Source: CAD feature listing. Evaluate the final solid. Frame: model axes, mm. Face numbers are marked on the shaded views. A direction names the side the tool comes from. Give positions to 0.01 mm unless a question says otherwise; leave off trailing zeros. Write each loop counter-clockwise with the first axis right and the second up, starting at its lowest first coordinate (ties: lowest second). Pieces come first, ordered by that corner, then holes. Notation, with made-up numbers: (87, -40) -> (121, -40) arc R15 ccw to (121, -17) -> close; hole circle Ø2 at (-12, -4.75). An arc over 180 degrees is marked (long way). Use a Markdown table: item, result. Add a question column.
```python
from build123d import *

# Parameters (mm, degrees)
EXTRUDE_1_DEPTH      = 7.5
EXTRUDE_1_DEPTH_BACK = 7.5
SKETCH_1_W           = 60
SKETCH_1_H           = 15
SKETCH_2_W           = 3
SKETCH_2_H           = 3
EXTRUDE_2_DEPTH      = 1
EXTRUDE_3_DEPTH      = 1
EXTRUDE_3_DEPTH_BACK = 4
CUT_EXTRUDE_1_REACH  = 36.667
SKETCH_5_W           = 54.5
SKETCH_5_H           = 13
CUT_EXTRUDE_2_DEPTH  = 13
CUT_EXTRUDE_3_DEPTH  = 9.45
EXTRUDE_4_REACH      = 40.81
SKETCH_7_W           = 0.3
SKETCH_7_H           = 6.5
CUT_EXTRUDE_4_REACH  = 40.082
CUT_EXTRUDE_5_REACH  = 37.798
FILLET_1_R           = 0.1
FILLET_2_R           = 0.2


with BuildPart() as part:
    # Sketch 1 → Extrude 1 (new, two sides: drawn at the far end of the back side and taken through both)
    with BuildSketch(Plane.XY.offset(-EXTRUDE_1_DEPTH_BACK)):
        with Locations((0, 7.5)):
            Rectangle(SKETCH_1_W, SKETCH_1_H)
    extrude(amount=EXTRUDE_1_DEPTH + EXTRUDE_1_DEPTH_BACK)

    # Sketch 2 → Extrude 2 (add)
    with BuildSketch(Plane(origin=(30, 0, 0), x_dir=(0, 0, -1), z_dir=(1, 0, 0))):
        with Locations((0, 7.5)):
            Rectangle(SKETCH_2_W, SKETCH_2_H)
    extrude(amount=EXTRUDE_2_DEPTH)

    # Sketch 3 → Extrude 3 (add, two sides: drawn at the far end of the back side and taken through both)
    with BuildSketch(Plane.XY.offset(1.5).offset(-EXTRUDE_3_DEPTH_BACK)):
        with BuildLine():
            Line((32.5, 9.45), (32.5, 5.55))
            Line((32.5, 5.55), (31.555590279, 5.55))
            ThreePointArc((31.555590279, 5.55), (31.088161527, 5.719957697), (30.677124344, 6))
            Line((30.677124344, 6), (30.677124344, 9))
            ThreePointArc((30.677124344, 9), (31.088161527, 9.280042303), (31.555590279, 9.45))
            Line((31.555590279, 9.45), (32.5, 9.45))
        make_face()
    extrude(amount=EXTRUDE_3_DEPTH + EXTRUDE_3_DEPTH_BACK)

    # Sketch 4 → Cut-Extrude 1 (cut, up to next)
    with BuildSketch(Plane(origin=(0, 9.45, 0), x_dir=(-1, 0, 0), z_dir=(0, 1, 0)), mode=Mode.PRIVATE) as cut_extrude_1_sk1:
        with BuildLine():
            Line((-32.5, -1.95), (-31.555590279, -1.95))
            ThreePointArc((-31.555590279, -1.95), (-31.088161527, -1.780042303), (-30.677124344, -1.5))
            Line((-30.677124344, -1.5), (-30.677124344, -2.5))
            Line((-30.677124344, -2.5), (-32.5, -2.5))
            Line((-32.5, -2.5), (-32.5, -1.95))
        make_face()
    cut_extrude_1_tool1 = extrude(cut_extrude_1_sk1.sketch, amount=-CUT_EXTRUDE_1_REACH, mode=Mode.PRIVATE) & part.part
    # Sketch 4 → Cut-Extrude 1 (cut, up to next)
    with BuildSketch(Plane(origin=(0, 9.45, 0), x_dir=(-1, 0, 0), z_dir=(0, 1, 0)), mode=Mode.PRIVATE) as cut_extrude_1_sk2:
        with BuildLine():
            Line((-30.677124344, 2.5), (-32.5, 2.5))
            Line((-32.5, 2.5), (-32.5, 1.95))
            Line((-32.5, 1.95), (-31.555590279, 1.95))
            ThreePointArc((-31.555590279, 1.95), (-31.088161527, 1.780042303), (-30.677124344, 1.5))
            Line((-30.677124344, 1.5), (-30.677124344, 2.5))
        make_face()
    cut_extrude_1_tool2 = extrude(cut_extrude_1_sk2.sketch, amount=-CUT_EXTRUDE_1_REACH, mode=Mode.PRIVATE) & part.part
    add(cut_extrude_1_tool1.solids().sort_by_distance((31.500125, 9.45, -2.169375))[0], mode=Mode.SUBTRACT)
    add(cut_extrude_1_tool2.solids().sort_by_distance((31.500125, 9.45, 2.169375))[0], mode=Mode.SUBTRACT)

    # Sketch 5 → Cut-Extrude 2 (cut)
    with BuildSketch(Plane.XY.offset(7.5)):
        with Locations((0.75, 8.5)):
            Rectangle(SKETCH_5_W, SKETCH_5_H)
    extrude(amount=-CUT_EXTRUDE_2_DEPTH, mode=Mode.SUBTRACT)

    # Sketch 6 → Cut-Extrude 3 (cut)
    with BuildSketch(Plane.XY.offset(7.5)):
        with BuildLine():
            Line((-27.2, 9.45), (-27.2, 5.55))
            Line((-27.2, 5.55), (-28.444409721, 5.55))
            ThreePointArc((-28.444409721, 5.55), (-28.911838473, 5.719957697), (-29.322875656, 6))
            Line((-29.322875656, 6), (-30, 6))
            Line((-30, 6), (-30, 9))
            Line((-30, 9), (-29.322875656, 9))
            ThreePointArc((-29.322875656, 9), (-28.911838473, 9.280042303), (-28.444409721, 9.45))
            Line((-28.444409721, 9.45), (-27.2, 9.45))
        make_face()
    extrude(amount=-CUT_EXTRUDE_3_DEPTH, mode=Mode.SUBTRACT)

    # Sketch 7 → Extrude 4 (add, up to next)
    with BuildSketch(Plane.XY.offset(7.5), mode=Mode.PRIVATE) as extrude_4_sk1:
        with Locations((-26.35, 7.5)):
            Rectangle(SKETCH_7_W, SKETCH_7_H)
    extrude_4_tool1 = extrude(extrude_4_sk1.sketch, amount=-EXTRUDE_4_REACH, mode=Mode.PRIVATE) - part.part
    add(extrude_4_tool1.solids().sort_by_distance((-26.35, 7.5, 7.5))[0])

    # Sketch 8 → Cut-Extrude 4 (cut, up to next)
    with BuildSketch(Plane.XY.offset(-5.5), mode=Mode.PRIVATE) as cut_extrude_4_sk1:
        with BuildLine():
            Line((-21.177124344, 9), (-19.25, 9))
            Line((-19.25, 9), (-19.25, 6))
            Line((-19.25, 6), (-21.177124344, 6))
            ThreePointArc((-21.177124344, 6), (-22.5, 5.5), (-23.822875656, 6))
            Line((-23.822875656, 6), (-25.75, 6))
            Line((-25.75, 6), (-25.75, 9))
            Line((-25.75, 9), (-23.822875656, 9))
            ThreePointArc((-23.822875656, 9), (-22.5, 9.5), (-21.177124344, 9))
        make_face()
    cut_extrude_4_tool1 = extrude(cut_extrude_4_sk1.sketch, amount=-CUT_EXTRUDE_4_REACH, mode=Mode.PRIVATE) & part.part
    # Sketch 8 → Cut-Extrude 4 (cut, up to next)
    with BuildSketch(Plane.XY.offset(-5.5), mode=Mode.PRIVATE) as cut_extrude_4_sk2:
        with BuildLine():
            Line((-10.75, 9), (-8.822875656, 9))
            ThreePointArc((-8.822875656, 9), (-7.5, 9.5), (-6.177124344, 9))
            Line((-6.177124344, 9), (-4.25, 9))
            Line((-4.25, 9), (-4.25, 6))
            Line((-4.25, 6), (-6.177124344, 6))
            ThreePointArc((-6.177124344, 6), (-7.5, 5.5), (-8.822875656, 6))
            Line((-8.822875656, 6), (-10.75, 6))
            Line((-10.75, 6), (-10.75, 9))
        make_face()
    cut_extrude_4_tool2 = extrude(cut_extrude_4_sk2.sketch, amount=-CUT_EXTRUDE_4_REACH, mode=Mode.PRIVATE) & part.part
    # Sketch 8 → Cut-Extrude 4 (cut, up to next)
    with BuildSketch(Plane.XY.offset(-5.5), mode=Mode.PRIVATE) as cut_extrude_4_sk3:
        with BuildLine():
            Line((6.177124344, 6), (4.25, 6))
            Line((4.25, 6), (4.25, 9))
            Line((4.25, 9), (6.177124344, 9))
            ThreePointArc((6.177124344, 9), (7.5, 9.5), (8.822875656, 9))
            Line((8.822875656, 9), (10.75, 9))
            Line((10.75, 9), (10.75, 6))
            Line((10.75, 6), (8.822875656, 6))
            ThreePointArc((8.822875656, 6), (7.5, 5.5), (6.177124344, 6))
        make_face()
    cut_extrude_4_tool3 = extrude(cut_extrude_4_sk3.sketch, amount=-CUT_EXTRUDE_4_REACH, mode=Mode.PRIVATE) & part.part
    # Sketch 8 → Cut-Extrude 4 (cut, up to next)
    with BuildSketch(Plane.XY.offset(-5.5), mode=Mode.PRIVATE) as cut_extrude_4_sk4:
        with BuildLine():
            Line((21.177124344, 6), (19.25, 6))
            Line((19.25, 6), (19.25, 9))
            Line((19.25, 9), (21.177124344, 9))
            ThreePointArc((21.177124344, 9), (22.5, 9.5), (23.822875656, 9))
            Line((23.822875656, 9), (25.75, 9))
            Line((25.75, 9), (25.75, 6))
            Line((25.75, 6), (23.822875656, 6))
            ThreePointArc((23.822875656, 6), (22.5, 5.5), (21.177124344, 6))
        make_face()
    cut_extrude_4_tool4 = extrude(cut_extrude_4_sk4.sketch, amount=-CUT_EXTRUDE_4_REACH, mode=Mode.PRIVATE) & part.part
    add(cut_extrude_4_tool1.solids().sort_by_distance((-22.5, 7.5, -5.5))[0], mode=Mode.SUBTRACT)
    add(cut_extrude_4_tool2.solids().sort_by_distance((-7.5, 7.5, -5.5))[0], mode=Mode.SUBTRACT)
    add(cut_extrude_4_tool3.solids().sort_by_distance((7.5, 7.5, -5.5))[0], mode=Mode.SUBTRACT)
    add(cut_extrude_4_tool4.solids().sort_by_distance((22.5, 7.5, -5.5))[0], mode=Mode.SUBTRACT)

    # Sketch 9 → Cut-Extrude 5 (cut, up to next)
    with BuildSketch(Plane(origin=(0, 2, 0), x_dir=(-1, 0, 0), z_dir=(0, 1, 0)), mode=Mode.PRIVATE) as cut_extrude_5_sk1:
        with BuildLine():
            Line((21.177124344, -1.5), (19.25, -1.5))
            Line((19.25, -1.5), (19.25, 1.5))
            Line((19.25, 1.5), (21.177124344, 1.5))
            ThreePointArc((21.177124344, 1.5), (22.5, 2), (23.822875656, 1.5))
            Line((23.822875656, 1.5), (25.75, 1.5))
            Line((25.75, 1.5), (25.75, -1.5))
            Line((25.75, -1.5), (23.822875656, -1.5))
            ThreePointArc((23.822875656, -1.5), (22.5, -2), (21.177124344, -1.5))
        make_face()
    cut_extrude_5_tool1 = extrude(cut_extrude_5_sk1.sketch, amount=-CUT_EXTRUDE_5_REACH, mode=Mode.PRIVATE) & part.part
    # Sketch 9 → Cut-Extrude 5 (cut, up to next)
    with BuildSketch(Plane(origin=(0, 2, 0), x_dir=(-1, 0, 0), z_dir=(0, 1, 0)), mode=Mode.PRIVATE) as cut_extrude_5_sk2:
        with BuildLine():
            Line((10.75, -1.5), (8.822875656, -1.5))
            ThreePointArc((8.822875656, -1.5), (7.5, -2), (6.177124344, -1.5))
            Line((6.177124344, -1.5), (4.25, -1.5))
            Line((4.25, -1.5), (4.25, 1.5))
            Line((4.25, 1.5), (6.177124344, 1.5))
            ThreePointArc((6.177124344, 1.5), (7.5, 2), (8.822875656, 1.5))
            Line((8.822875656, 1.5), (10.75, 1.5))
            Line((10.75, 1.5), (10.75, -1.5))
        make_face()
    cut_extrude_5_tool2 = extrude(cut_extrude_5_sk2.sketch, amount=-CUT_EXTRUDE_5_REACH, mode=Mode.PRIVATE) & part.part
    # Sketch 9 → Cut-Extrude 5 (cut, up to next)
    with BuildSketch(Plane(origin=(0, 2, 0), x_dir=(-1, 0, 0), z_dir=(0, 1, 0)), mode=Mode.PRIVATE) as cut_extrude_5_sk3:
        with BuildLine():
            Line((-6.177124344, 1.5), (-4.25, 1.5))
            Line((-4.25, 1.5), (-4.25, -1.5))
            Line((-4.25, -1.5), (-6.177124344, -1.5))
            ThreePointArc((-6.177124344, -1.5), (-7.5, -2), (-8.822875656, -1.5))
            Line((-8.822875656, -1.5), (-10.75, -1.5))
            Line((-10.75, -1.5), (-10.75, 1.5))
            Line((-10.75, 1.5), (-8.822875656, 1.5))
            ThreePointArc((-8.822875656, 1.5), (-7.5, 2), (-6.177124344, 1.5))
        make_face()
    cut_extrude_5_tool3 = extrude(cut_extrude_5_sk3.sketch, amount=-CUT_EXTRUDE_5_REACH, mode=Mode.PRIVATE) & part.part
    # Sketch 9 → Cut-Extrude 5 (cut, up to next)
    with BuildSketch(Plane(origin=(0, 2, 0), x_dir=(-1, 0, 0), z_dir=(0, 1, 0)), mode=Mode.PRIVATE) as cut_extrude_5_sk4:
        with BuildLine():
            Line((-21.177124344, 1.5), (-19.25, 1.5))
            Line((-19.25, 1.5), (-19.25, -1.5))
            Line((-19.25, -1.5), (-21.177124344, -1.5))
            ThreePointArc((-21.177124344, -1.5), (-22.5, -2), (-23.822875656, -1.5))
            Line((-23.822875656, -1.5), (-25.75, -1.5))
            Line((-25.75, -1.5), (-25.75, 1.5))
            Line((-25.75, 1.5), (-23.822875656, 1.5))
            ThreePointArc((-23.822875656, 1.5), (-22.5, 2), (-21.177124344, 1.5))
        make_face()
    cut_extrude_5_tool4 = extrude(cut_extrude_5_sk4.sketch, amount=-CUT_EXTRUDE_5_REACH, mode=Mode.PRIVATE) & part.part
    add(cut_extrude_5_tool1.solids().sort_by_distance((-22.5, 2, 0))[0], mode=Mode.SUBTRACT)
    add(cut_extrude_5_tool2.solids().sort_by_distance((-7.5, 2, 0))[0], mode=Mode.SUBTRACT)
    add(cut_extrude_5_tool3.solids().sort_by_distance((7.5, 2, 0))[0], mode=Mode.SUBTRACT)
    add(cut_extrude_5_tool4.solids().sort_by_distance((22.5, 2, 0))[0], mode=Mode.SUBTRACT)

    # Fillet 1
    fillet_1_edges = [part.edges().sort_by_distance(p)[0] for p in [
        (32.5, 5.55, 0),
        (32.5, 9.45, 0),
        (32.5, 7.5, -1.95),
        (32.5, 7.5, 1.95),
    ]]
    fillet(fillet_1_edges, radius=FILLET_1_R)

    # Fillet 2
    fillet_2_edges = [part.edges().sort_by_distance(p)[0] for p in [
        (-30, 3, 7.5),
        (-30, 0, 0),
        (-30, 7.5, -7.5),
        (-30, 15, 0),
        (-30, 12, 7.5),
        (-30, 9, 2.775),
        (-30, 7.5, -1.95),
        (-30, 6, 2.775),
        (0, 0, -7.5),
        (0, 0, 7.5),
        (0, 15, -7.5),
        (30, 0, 0),
        (30, 7.5, -7.5),
        (30, 15, 0),
        (29, 15, 7.5),
        (30, 7.5, 7.5),
    ]]
    fillet(fillet_2_edges, radius=FILLET_2_R)


solid = part.part
```
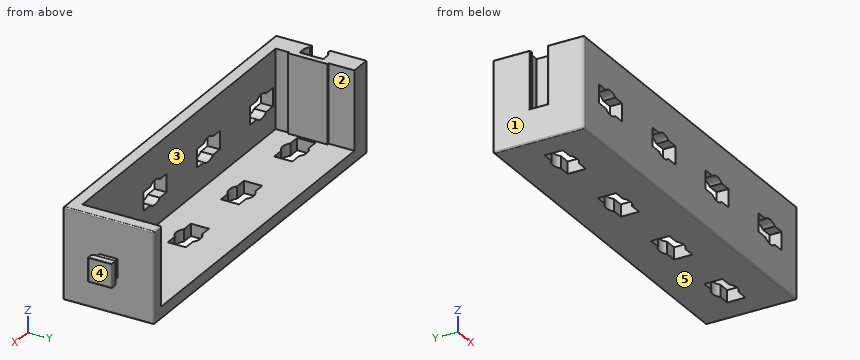
(1) Material intervals for L1, parallel to X at y = 8.25, z = -5.75; L2, parallel to X at y = 5.5, z = 4.25; L3, parallel to X at y = 11, z = 1.75, sorted ascending.
(2) Cut plane C-C on y = 12.5. Return the cut outline in (x, z), then the cut area to 3 significant figures.
(3) First-contact query: pin 1 Ø6 at (y, z) = (7, 2) entering from +X; pin 2 Ø4 at (y, z) = (12.5, -0.5) entering from +X; pin 3 Ø1 at (x, y) = (1, 4.5) entering from +Z. Flat tips, straight axial feed; report the tip coordinate or a pass-through.
(4) Cut plane B-B on z = 3.25. Return the cut outline in (x, y).
(5) Access query for the marked faces 1 and 2. Directions: +Z, -Z, +X, -X, +Y, -Y. A direction counts if a zero-diameter tool reaches every point of the face in a straight line with its end or side. Return the directions, or none.
(6) Mould query, pull axis X, two halves, no side actions, for the marked faces 3, 4 and 5. Classes: +X half, -X half, draft (parallel to the pull), parting line (faces both ways), or undercut.
(7) Cut plane A-A on x = -20. Return the cut outline in (y, z), then the cut area to 3 significant figures.
(8) Cut plane D-D on y = 6.75. Count the separate pieces of the cut face and the enclosed holes in it, then the cut area to 3 significant figures.
Output:
| question | item | result |
|---|---|---|
| 1 | L1 | -30 to -25.75, -19.25 to -10.75, -4.25 to 4.25, 10.75 to 19.25, 25.75 to 30 |
| 1 | L2 | -30 to -26.2, 28 to 30 |
| 1 | L3 | -30 to -26.5, 28 to 30 |
| 2 | outline | (-30, -7.3) arc R0.2 ccw to (-29.8, -7.5) -> (29.8, -7.5) arc R0.2 ccw to (30, -7.3) -> (30, 7.3) arc R0.2 ccw to (29.8, 7.5) -> (28, 7.5) -> (28, -5.5) -> (-26.5, -5.5) -> (-26.5, 7.5) -> (-29.8, 7.5) arc R0.2 ccw to (-30, 7.3) -> close |
| 2 | area | 191 mm^2 |
| 3 | pin 1 | x = 32.5 |
| 3 | pin 2 | x = 30 |
| 3 | pin 3 | z = -5.5 |
| 4 | outline | (-30, 0.2) arc R0.2 ccw to (-29.8, 0) -> (29.8, 0) arc R0.2 ccw to (30, 0.2) -> (30, 14.8) arc R0.2 ccw to (29.8, 15) -> (28, 15) -> (28, 2) -> (-26.5, 2) -> (-26.5, 4.25) -> (-26.2, 4.25) -> (-26.2, 10.75) -> (-26.5, 10.75) -> (-26.5, 15) -> (-29.8, 15) arc R0.2 ccw to (-30, 14.8) -> (-30, 9.2) arc R0.2 ccw to (-29.8, 9) -> (-29.32, 9) arc R2 cw to (-28.44, 9.45) -> (-27.2, 9.45) -> (-27.2, 5.55) -> (-28.44, 5.55) arc R2 cw to (-29.32, 6) -> (-29.8, 6) arc R0.2 ccw to (-30, 5.8) -> close |
| 5 | face 1 | +Z, -Z, -X, +Y, -Y |
| 5 | face 2 | +Z, +Y |
| 6 | face 3 | undercut |
| 6 | face 4 | +X half |
| 6 | face 5 | draft |
| 7 | outline | (0, -7.3) arc R0.2 ccw to (0.2, -7.5) -> (6, -7.5) -> (6, -5.5) -> (2, -5.5) -> (2, -1.5) -> (0, -1.5) -> close; (0, 1.5) -> (2, 1.5) -> (2, 7.5) -> (0.2, 7.5) arc R0.2 ccw to (0, 7.3) -> close; (9, -7.5) -> (14.8, -7.5) arc R0.2 ccw to (15, -7.3) -> (15, -5.5) -> (9, -5.5) -> close |
| 7 | area | 44.0 mm^2 |
| 8 | separate pieces | 5 |
| 8 | enclosed holes | 0 |
| 8 | area | 126 mm^2 |
